Input: part model. Units: mm. Frame: model coordinates. Coordinates: 2 decimals unless noted, no trailing zeros. Write each loop counter-clockwise with the first axis right and the second up, starting at its lowest first coordinate (ties: lowest second). Pieces come first, ordered by that corner, then holes.
1) Section query A-A (y = -11.5). Output: boundary loops of the cut face in (x, z) (1 decimal), then the cut area to 3 significant figures.
2) Line query: L1, parallel to Y at x = -43, z = 0.65 (3 decimals); L2, parallel to Y at x = -6, z = 1.7 (3 decimals); L3, parallel to X at y = -36, z = 0.55. Output: solid intervals per line, ascending.
3) Section query B-B (z = 1.3). State how many separate pieces and enclosed holes the cut face has, then the cut area to 3 significant figures.
4) Pin query (flat end, axial travel): pin 1 Ø1.9 at (x, y) = (-80.96, 38.1) entering from -Z; pin 2 Ø5 at (x, y) = (-23.81, -19.05) entering from -Z. Return the tip coordinate at first contact, or that it passes through.
Autodesk Inventor part; units mm, degrees
ref_plane "YZ Plane" through (0, 0, 0) normal (1, 0, 0) x (0, 1, 0)
ref_plane "XZ Plane" through (0, 0, 0) normal (0, 1, 0) x (-1, 0, 0)
ref_plane "XY Plane" through (0, 0, 0) normal (0, 0, 1) x (1, 0, 0)
sketch "Sketch1" plane through (0, 0, 0) normal (0, 0, 1) x (1, 0, 0)
  line L0 (-188.9125, -66.675) -> (188.9125, -66.675)
  line L1 (188.9125, -66.675) -> (188.9125, 66.675)
  line L2 (188.9125, 66.675) -> (-188.9125, 66.675)
  line L3 (-188.9125, 66.675) -> (-188.9125, -66.675)
  line L4 (-188.9125, -66.675) -> (188.9125, 66.675) construction
  line L5 (188.9125, -66.675) -> (-188.9125, 66.675) construction
  point P0 (0, 0)
  dimension "d0" = 133.35
  dimension "d1" = 377.825
extrude "Extrusion1" add sketch "Sketch1" along normal blind 3.175
sketch "Sketch2" plane through (0, 0, 3.175) normal (0, 0, 1) x (1, 0, 0)
  line L0 (-138.1125, -41.275) -> (87.3125, -41.275)
  line L1 (87.3125, -41.275) -> (87.3125, 41.275)
  line L2 (87.3125, 41.275) -> (-138.1125, 41.275)
  line L3 (-138.1125, 41.275) -> (-138.1125, -41.275)
  line L4 (-188.9125, -66.675) -> (188.9125, -66.675)
  line L5 (188.9125, 66.675) -> (-188.9125, 66.675)
  line L6 (-188.9125, 66.675) -> (-188.9125, -66.675)
  line L7 (188.9125, -66.675) -> (188.9125, 66.675)
  point P0 (0, 0)
  point P1 (-138.1125, 19.05)
  point P2 (-138.1125, -19.05)
  point P3 (-138.1125, 0)
  point P4 (-119.0625, 19.05)
  point P5 (-119.0625, 0)
  point P6 (-119.0625, -19.05)
  point P7 (-100.0125, 19.05)
  point P8 (-100.0125, 0)
  point P9 (-100.0125, -19.05)
  point P10 (-80.9625, 19.05)
  point P11 (-80.9625, 0)
  point P12 (-80.9625, -19.05)
  point P13 (-61.9125, 19.05)
  point P14 (-61.9125, 0)
  point P15 (-61.9125, -19.05)
  point P16 (-42.8625, 19.05)
  point P17 (-42.8625, 0)
  point P18 (-42.8625, -19.05)
  point P19 (-23.8125, 19.05)
  point P20 (-23.8125, 0)
  point P21 (-23.8125, -19.05)
  point P22 (-4.7625, 19.05)
  point P23 (-4.7625, 0)
  point P24 (-4.7625, -19.05)
  point P25 (14.2875, 19.05)
  point P26 (14.2875, 0)
  point P27 (14.2875, -19.05)
  point P28 (33.3375, 19.05)
  point P29 (33.3375, 0)
  point P30 (33.3375, -19.05)
  point P31 (52.3875, 19.05)
  point P32 (52.3875, 0)
  point P33 (52.3875, -19.05)
  point P34 (71.4375, 19.05)
  point P35 (71.4375, 0)
  point P36 (71.4375, -19.05)
  point P37 (90.4875, 19.05)
  point P38 (90.4875, 0)
  point P39 (90.4875, -19.05)
  point P40 (-138.1125, -38.1)
  point P41 (-119.0625, -38.1)
  point P42 (-100.0125, -38.1)
  point P43 (-80.9625, -38.1)
  point P44 (-61.9125, -38.1)
  point P45 (-42.8625, -38.1)
  point P46 (-23.8125, -38.1)
  point P47 (-4.7625, -38.1)
  point P48 (14.2875, -38.1)
  point P49 (33.3375, -38.1)
  point P50 (52.3875, -38.1)
  point P51 (71.4375, -38.1)
  point P52 (90.4875, -38.1)
  point P53 (90.4875, 38.1)
  point P54 (71.4375, 38.1)
  point P55 (52.3875, 38.1)
  point P56 (33.3375, 38.1)
  point P57 (14.2875, 38.1)
  point P58 (-4.7625, 38.1)
  point P59 (-23.8125, 38.1)
  point P60 (-42.8625, 38.1)
  point P61 (-61.9125, 38.1)
  point P62 (-80.9625, 38.1)
  point P63 (-100.0125, 38.1)
  point P64 (-119.0625, 38.1)
  point P65 (-138.1125, 38.1)
  dimension "d4" = 25.4
  dimension "d5" = 25.4
  dimension "d6" = 50.8
  dimension "d7" = 101.6
  dimension "d8" = 22.225
  dimension "d9" = 0
  dimension "d10" = 22.225
  dimension "d13" = 19.05
  dimension "d33" = 19.05
  dimension "d40" = 19.05
hole "Hole1" at (-138.1125, 19.05, 3.175) at (-138.1125, -19.05, 3.175) at (-138.1125, 0, 3.175) at (-119.0625, 19.05, 3.175) at (-119.0625, 0, 3.175) at (-119.0625, -19.05, 3.175) at (-100.0125, 19.05, 3.175) at (-100.0125, 0, 3.175) at (-100.0125, -19.05, 3.175) at (-80.9625, 19.05, 3.175) at (-80.9625, 0, 3.175) at (-80.9625, -19.05, 3.175) at (-61.9125, 19.05, 3.175) at (-61.9125, 0, 3.175) at (-61.9125, -19.05, 3.175) at (-42.8625, 19.05, 3.175) at (-42.8625, 0, 3.175) at (-42.8625, -19.05, 3.175) at (-23.8125, 19.05, 3.175) at (-23.8125, 0, 3.175) at (-23.8125, -19.05, 3.175) at (-4.7625, 19.05, 3.175) at (-4.7625, 0, 3.175) at (-4.7625, -19.05, 3.175) at (14.2875, 19.05, 3.175) at (14.2875, 0, 3.175) at (14.2875, -19.05, 3.175) at (33.3375, 19.05, 3.175) at (33.3375, 0, 3.175) at (33.3375, -19.05, 3.175) at (52.3875, 19.05, 3.175) at (52.3875, 0, 3.175) at (52.3875, -19.05, 3.175) at (71.4375, 19.05, 3.175) at (71.4375, 0, 3.175) at (71.4375, -19.05, 3.175) at (90.4875, 19.05, 3.175) at (90.4875, 0, 3.175) at (90.4875, -19.05, 3.175) direction (0, 0, -1) diameter 3.175 end through all
sketch "Sketch4" plane through (0, 0, 3.175) normal (0, 0, 1) x (1, 0, 0)
  line L0 (179.3875, 44.45) -> (144.4625, 44.45)
  line L1 (144.4625, 44.45) -> (144.4625, -44.45)
  line L2 (144.4625, -44.45) -> (179.3875, -44.45)
  line L3 (179.3875, -44.45) -> (179.3875, 44.45)
  line L4 (188.9125, -66.675) -> (188.9125, 66.675)
  line L5 (188.9125, 66.675) -> (-188.9125, 66.675)
  line L6 (-188.9125, -66.675) -> (188.9125, -66.675)
  point P0 (0, 0)
  dimension "d25" = 9.525
  dimension "d26" = 44.45
  dimension "d27" = 22.225
  dimension "d28" = 22.225
extrude "Extrusion2" cut sketch "Sketch4" against normal blind 25.4
hole "Hole2" at (-138.1125, -38.1, 3.175) at (-119.0625, -38.1, 3.175) at (-100.0125, -38.1, 3.175) at (-80.9625, -38.1, 3.175) at (-61.9125, -38.1, 3.175) at (-42.8625, -38.1, 3.175) at (-23.8125, -38.1, 3.175) at (-4.7625, -38.1, 3.175) at (14.2875, -38.1, 3.175) at (33.3375, -38.1, 3.175) at (52.3875, -38.1, 3.175) at (71.4375, -38.1, 3.175) at (90.4875, -38.1, 3.175) at (90.4875, 38.1, 3.175) at (71.4375, 38.1, 3.175) at (52.3875, 38.1, 3.175) at (33.3375, 38.1, 3.175) at (14.2875, 38.1, 3.175) at (-4.7625, 38.1, 3.175) at (-23.8125, 38.1, 3.175) at (-42.8625, 38.1, 3.175) at (-61.9125, 38.1, 3.175) at (-80.9625, 38.1, 3.175) at (-100.0125, 38.1, 3.175) at (-119.0625, 38.1, 3.175) at (-138.1125, 38.1, 3.175) direction (0, 0, -1) diameter 3.175 end through all
properties part number "perforated side"
Answer:
1. outline: (-188.9, 0) - (144.5, 0) - (144.5, 3.2) - (-188.9, 3.2) - close; (179.4, 0) - (188.9, 0) - (188.9, 3.2) - (179.4, 3.2) - close
1. area: 1,090 mm2
2. L1: y = -66.675 to -39.682, -36.518 to -20.632, -17.468 to -1.582, 1.582 to 17.468, 20.632 to 36.518, 39.682 to 66.675
2. L2: y = -66.675 to -39.094, -37.106 to -20.044, -18.056 to -0.994, 0.994 to 18.056, 20.044 to 37.106, 39.094 to 66.675
2. L3: x = -188.91 to 144.46, 179.39 to 188.91
3. separate pieces: 1
3. enclosed holes: 66
3. area: 46,800 mm2
4. pin 1: passes through
4. pin 2: stops at z = 0
